Solid Edge part; units mm, degrees
sketch "Sketch1" plane through (0, 0, 0) normal (0, -1, 0) x (1, 0, 0)
  line L0 (0, 22.6935) -> (0, -22.6935)
  arc A0 (0, 22.6935) -> (0, -22.6935) centre (0, 0) cw
revolve "RevolvedProtrusion1" add sketch "Sketch1" angle 360 about axis through (0, 0, 22.6935) along (0, 0, -1)
sketch "Sketch2" plane through (0, 0, 0) normal (0, 0, 1) x (1, 0, 0)
  circle A0 centre (0, 0) radius 45.712
extrude "Protrusion1" add sketch "Sketch2" along normal mid plane 2.35
sketch "Sketch3" plane through (0, 0, 0) normal (0, 0, 1) x (1, 0, 0)
  circle A0 centre (0, 0) radius 31.7083
extrude "ExtrudedProtrusion_9" add sketch "Sketch3" along normal mid plane 2.36
sketch "Sketch4" plane through (0, 0, 0) normal (0, 0, 1) x (1, 0, 0)
  circle A0 centre (0, 0) radius 5.09
extrude "ExtrudedCutout_1" cut sketch "Sketch4" against normal blind 53.2556
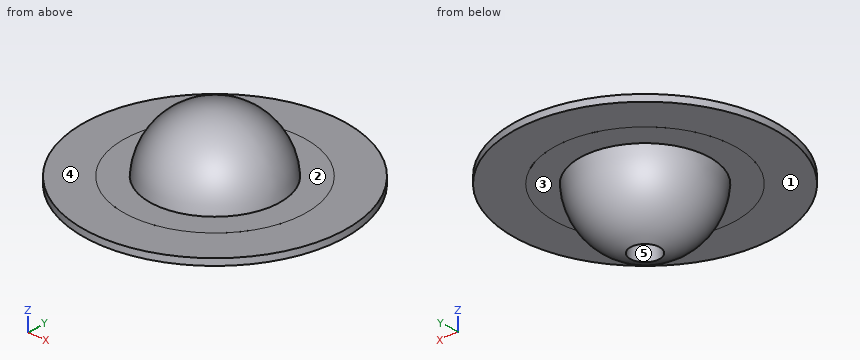
The listing builds one solid part. Answer for the finished solid, in the listing's coordinates (mm). Face numbers are marked on the shaded views. A direction names the side the tool comes from. Give positions to 0.01 mm unless a question says otherwise; leave off trailing zeros. Write each loop counter-clockwise with the first axis right and the second up, starting at its lowest first coordinate (ties: lowest second). Pieces come first, ordered by that corner, then holes. Notation, with made-up numbers: (51, 26) - (103, 26) arc R20 cw to (103, 64) - close; hole circle Ø10 at (-5.5, 37). An arc over 180 degrees is marked (long way). Use a Markdown table: item, result.
1. Each of these flat-tipped pins is pushed along its axis until it touches: P1, Ø1, axis at x = -29, z = 3.5, coming from the -Y side; P2, Ø1.5, axis at y = 2.5, z = -7.5, coming from the -X side; P3, Ø12, axis at x = 22, y = -34, coming from the -Z side (3 decimals); P4, Ø3, axis at x = -5, z = -3.5, coming from the +Y side. Where does it stop, or does it pass through?
Values follow:
| item | result |
|---|---|
| P1 | passes through |
| P2 | stops at x = -21.54 |
| P3 | stops at z = -1.175 |
| P4 | stops at y = 22.22 |
2. Section D-D on y = 21.5 is taken. Write down the section's boundary in (x, z) (3 decimals), plus the area to 3 significant figures.
Values follow:
| item | result |
|---|---|
| outline | (-40.34, -1.175) - (-23.306, -1.175) - (-23.306, -1.18) - (-7.166, -1.18) arc R7.263 ccw to (7.166, -1.18) - (23.306, -1.18) - (23.306, -1.175) - (40.34, -1.175) - (40.34, 1.175) - (23.306, 1.175) - (23.306, 1.18) - (7.166, 1.18) arc R7.263 ccw to (-7.166, 1.18) - (-23.306, 1.18) - (-23.306, 1.175) - (-40.34, 1.175) - close |
| area | 322 mm² |
3. For a pull along Z with two mould halves and no side action, classify the marked faces 3, 4 and 5 as released by +Z, released by -Z, zero draft, split by the parting line, or undercut.
Values follow:
| item | result |
|---|---|
| face 3 | released by -Z |
| face 4 | released by +Z |
| face 5 | zero draft |
4. A tool of negligible diameter and unlimited length cuts with its end or side. For the marked faces 1 and 2, from which of +Z, -Z, +X, -X, +Y, -Y can it reach the whole face along a straight path? Write none if from no direction.
Values follow:
| item | result |
|---|---|
| face 1 | -Z |
| face 2 | +Z |
5. Section C-C on z = -3 is taken. Write down the section's boundary in (x, y), plus the area to 3 significant figures.
Values follow:
| item | result |
|---|---|
| outline | circle Ø44.99 at (0, 0); hole circle Ø10.18 at (0, 0) |
| area | 1,510 mm² |
6. Find the intervals of material crossed by probe 1 along Z at (x, y) = (-4, -37) (3 decimals); probe 2 along Y at (x, z) = (0, -4.25); probe 3 along Y at (x, z) = (0, -15), in increasing order. Write a range as from..to.
Values follow:
| item | result |
|---|---|
| probe 1 | z = -1.175..1.175 |
| probe 2 | y = -22.29..-5.09, 5.09..22.29 |
| probe 3 | y = -17.03..-5.09, 5.09..17.03 |
